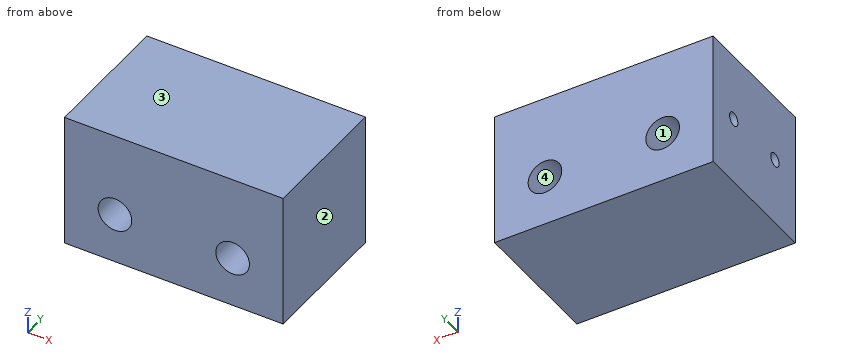
from build123d import *

# Parameters (mm, degrees)
SKETCH1_W                   = 82.55
SKETCH1_H                   = 50.8
BOSS_EXTRUDE1_DEPTH         = 25.4
F_1_2_0_5000_DOWEL_HOLE1_D  = 12.7
F_1_4_20_TAPPED_HOLE1_D     = 5.1054
F_1_4_20_TAPPED_HOLE1_DEPTH = 12.7
F_1_4_20_TAPPED_HOLE1_TIP   = 1.533816902


with BuildPart() as part:
    # Sketch1 → Boss-Extrude1 (new, symmetric)
    with BuildSketch(Plane(origin=(0, 0, 0), x_dir=(1, 0, 0), z_dir=(0, 1, 0))):
        Rectangle(SKETCH1_W, SKETCH1_H)
    extrude(amount=BOSS_EXTRUDE1_DEPTH, both=True)

    # 1/2 (0.5000) Dowel Hole1 (through all)
    with Locations(Plane(origin=(0, 25.4, 0), x_dir=(1, 0, 0), z_dir=(0, 1, 0))):
        with Locations((22.225, 6.35), (-22.225, 6.35)):
            Hole(F_1_2_0_5000_DOWEL_HOLE1_D / 2)

    # 1/4-20 Tapped Hole1
    with Locations(Plane.ZY.offset(41.275)):
        with Locations((0, 12.7), (0, -12.7)):
            Hole(F_1_4_20_TAPPED_HOLE1_D / 2, depth=F_1_4_20_TAPPED_HOLE1_DEPTH)
            with Locations((0, 0, -(F_1_4_20_TAPPED_HOLE1_DEPTH + F_1_4_20_TAPPED_HOLE1_TIP / 2))):  # 118° drill point
                Cone(0, F_1_4_20_TAPPED_HOLE1_D / 2, F_1_4_20_TAPPED_HOLE1_TIP, mode=Mode.SUBTRACT)


solid = part.part
Source: CAD feature listing. Evaluate the final solid. Frame: model axes, mm. Face numbers are marked on the shaded views. Give positions to 0.01 mm unless a question says otherwise; leave off trailing zeros. Write each loop counter-clockwise with the first axis right and the second up, starting at its lowest first coordinate (ties: lowest second). Pieces come first, ordered by that corner, then holes. Notation, with made-up numbers: M 54.5,83 L 102.5,83 A22 ccw 102.5,119 Z; hole C 26,10 d10. An arc over 180 degrees is marked long. Answer as a JSON object with one key per item and string values.
Q1. Cut plane A-A, the plane z = -6.35. Return the cut outline in (x, y) (3 decimals), then the cut area to 3 significant figures.
Geometry check:
{"outline": "M -41.275,-25.4 L -28.575,-25.4 L -28.575,25.4 L -41.275,25.4 Z; M -15.875,-25.4 L 15.875,-25.4 L 15.875,25.4 L -15.875,25.4 Z; M 28.575,-25.4 L 41.275,-25.4 L 41.275,25.4 L 28.575,25.4 Z", "area": "2,900 mm^2"}
Q2. Contact query for flat-ended pins moving along their axis: P1, Ø10, axis at x = 22.225, z = -6.35, coming from the +Y side; P2, Ø6, axis at y = 12.7, z = 0, coming from the -X side (3 decimals). Output: stop coordinate, or through.
Geometry check:
{"P1": "passes through", "P2": "stops at x = -41.275"}
Q3. Cut plane B-B, the plane x = 24. Return the cut outline in (y, z).
Geometry check:
{"outline": "M -25.4,-25.4 L 25.4,-25.4 L 25.4,-12.45 L -25.4,-12.45 Z; M -25.4,-0.25 L 25.4,-0.25 L 25.4,25.4 L -25.4,25.4 Z"}
Q4. Ray query, line 1 along Y through (x, z) = (-33, 0); line 2 along Z through (x, y) = (-33.25, -12.7); line 3 along X through (y, z) = (3, -6) (3 decimals). Return the intervals inside material, ascending.
Geometry check:
{"line 1": "y = -25.4 to -15.25, -10.15 to 10.15, 15.25 to 25.4", "line 2": "z = -25.4 to -2.55, 2.55 to 25.4", "line 3": "x = -41.275 to -28.565, -15.885 to 15.885, 28.565 to 41.275"}
Q5. Cut plane C-C, the plane y = 6. Return the cut outline in (x, z) (3 decimals).
Geometry check:
{"outline": "M -41.275,-25.4 L 41.275,-25.4 L 41.275,25.4 L -41.275,25.4 Z; hole C -22.225,-6.35 d12.7; hole C 22.225,-6.35 d12.7"}
Q6. Mould query, pull axis Z, two halves, no side actions, for the marked faces 1, 2, 3 and 4. Classes: +Z half, -Z half, draft (parallel to the pull), parting line (faces both ways), or undercut.
Geometry check:
{"face 1": "undercut", "face 2": "draft", "face 3": "+Z half", "face 4": "undercut"}
